For this review, take the finished solid that the model builds, in its own axes (mm). A direction names the side the tool comes from. Coordinates: 2 decimals unless noted, no trailing zeros. Loops run counter-clockwise (first coordinate to the right, second up) from the corner with the lowest first, then second, coordinate; pieces in that order, holes last. Notation, with made-up numbers: M -17.75,57.5 L 41.25,57.5 A21 cw 41.25,93.5 Z; hole C 44.5,14.5 d5. An arc over 180 degrees is marked long. Write item = value, one per line.
from build123d import *

# Parameters (mm, degrees)
F1_R          = 8.89
F1_R_2        = 5.969
F3_R          = 8.89
F3_R_2        = 7.62
F4_DEPTH      = 7.62
F5_DEPTH      = 25.4
F5_DEPTH_BACK = 25.4
F6_R          = 7.62
F7_R          = 7.62
F8_DEPTH      = 25.4
F0_W          = 25.4
F0_H          = 12.7
F9_DEPTH      = 8.89
F9_DEPTH_BACK = 8.89
F10_DEPTH     = 25.4


with BuildPart() as f2:
    # F2: sweep along a path in F0
    with BuildLine(Plane.XY) as f2_path:
        Line((0, 0), (0, 68.940756))
        ThreePointArc((0, 68.940756), (12.7, 81.640756), (25.4, 68.940756))
        Line((25.4, 68.940756), (25.4, 0))
    # F1 (on Front) → F2 (sweep)
    with BuildSketch(Plane.XZ):
        Circle(F1_R)
        Circle(F1_R_2, mode=Mode.SUBTRACT)
    sweep(path=f2_path.line)

    # F3 (on face) → F4 (cut)
    with BuildSketch(Plane.XZ):
        Circle(F3_R)
        Circle(F3_R_2, mode=Mode.SUBTRACT)
        with BuildLine():
            ThreePointArc((34.29, 0), (25.4, 8.89), (16.51, 0))
            ThreePointArc((16.51, 0), (25.4, -8.89), (34.29, 0))
        make_face()
        with BuildLine():
            ThreePointArc((33.02, 0), (25.4, -7.62), (17.78, 0))
            ThreePointArc((17.78, 0), (25.4, 7.62), (33.02, 0))
        make_face(mode=Mode.SUBTRACT)
    extrude(amount=-F4_DEPTH, mode=Mode.SUBTRACT)

    # F0 (on Top) → F5 (cut, two sides)
    with BuildSketch(Plane.XY) as f5_sk:
        with BuildLine():
            Line((-11.195335, 39.121766), (0, 39.121766))
            Line((0, 39.121766), (0, 68.940756))
            ThreePointArc((0, 68.940756), (3.719744, 77.921012), (12.7, 81.640756))
            ThreePointArc((12.7, 81.640756), (21.680256, 77.921012), (25.4, 68.940756))
            Line((25.4, 68.940756), (25.4, 39.121766))
            Line((25.4, 39.121766), (39.424099, 39.121766))
            Line((39.424099, 39.121766), (39.424099, 94.536379))
            Line((39.424099, 94.536379), (-11.195335, 94.536379))
            Line((-11.195335, 94.536379), (-11.195335, 39.121766))
        make_face()
        with BuildLine():
            Line((0, 68.940756), (0, 39.121766))
            Line((0, 39.121766), (12.7, 39.121766))
            Line((12.7, 39.121766), (12.7, 81.640756))
            ThreePointArc((12.7, 81.640756), (3.719744, 77.921012), (0, 68.940756))
        make_face()
        with BuildLine():
            Line((12.7, 39.121766), (25.4, 39.121766))
            Line((25.4, 39.121766), (25.4, 68.940756))
            ThreePointArc((25.4, 68.940756), (21.680256, 77.921012), (12.7, 81.640756))
            Line((12.7, 81.640756), (12.7, 39.121766))
        make_face()
    extrude(amount=F5_DEPTH, mode=Mode.SUBTRACT)
    extrude(f5_sk.sketch, amount=-F5_DEPTH_BACK, mode=Mode.SUBTRACT)

    # F6 (on face) + F7 (on face) → F8 (cut)
    with BuildSketch(Plane(origin=(0, 39.121766, 0), x_dir=(-1, 0, 0), z_dir=(0, 1, 0))):
        Circle(F6_R)
    with BuildSketch(Plane(origin=(0, 39.121766, 0), x_dir=(-1, 0, 0), z_dir=(0, 1, 0))):
        with Locations((-25.4, 0)):
            Circle(F7_R)
    extrude(amount=-F8_DEPTH, mode=Mode.SUBTRACT)

    # F0 (on Top) → F9 (join, two sides)
    with BuildSketch(Plane.XY) as f9_sk:
        with Locations((12.7, 26.517263)):
            Rectangle(F0_W, F0_H)
    extrude(amount=F9_DEPTH)
    extrude(f9_sk.sketch, amount=-F9_DEPTH_BACK)

    # F7 (on face) + F6 (on face) → F10 (cut)
    with BuildSketch(Plane(origin=(0, 39.121766, 0), x_dir=(-1, 0, 0), z_dir=(0, 1, 0))):
        with Locations((-25.4, 0)):
            Circle(F7_R)
    with BuildSketch(Plane(origin=(0, 39.121766, 0), x_dir=(-1, 0, 0), z_dir=(0, 1, 0))):
        Circle(F6_R)
    extrude(amount=-F10_DEPTH, mode=Mode.SUBTRACT)


solid = f2.part
Q1. For pin 1 Ø9 at (x, z) = (25.4, 0) entering from +Y; pin 2 Ø4.5 at (x, z) = (29, -2.5) entering from +Y; pin 3 Ø5 at (x, y) = (24.5, 4.5) entering from -Z; pin 4 Ø5.5 at (x, z) = (13.5, -4) entering from -Y, all flat-tipped, find the tip position at first contact; note any pin that passes through.
Solved:
pin_1 = through
pin_2 = 13.72
pin_3 = -7.62
pin_4 = 20.17
Q2. Draft analysis for pull direction Z (two halves, no side actions). For faces 1 (the face through (31.363, 6.765, -0.262)), 2 (the face through (33.013, 3.757, 0.335)), 3 (the face through (7, 39.122, 4)), state which applies: +Z half, -Z half, draft (parallel to the pull), parting line (faces both ways), or undercut.
Solved:
face_1 = undercut
face_2 = parting line
face_3 = draft
Q3. Add section B-B (x = 27.5). Write out the cut boundary in (y, z), and give its area (3 significant figures).
Solved:
outline = M 0,-7.32 L 7.62,-7.32 L 7.62,-8.64 L 39.12,-8.64 L 39.12,-7.32 L 13.72,-7.32 L 13.72,-5.59 L 0,-5.59 Z; M 0,5.59 L 13.72,5.59 L 13.72,7.32 L 39.12,7.32 L 39.12,8.64 L 7.62,8.64 L 7.62,7.32 L 0,7.32 Z
area = 130 mm²
Q4. For line 1 along Z through (x, y) = (25, 33); line 2 along X through (y, z) = (33, 3.5); line 3 along X through (y, z) = (21, 1.5), list the stretches that pass through material, from the lowest coordinate up.
Solved:
line_1 = -8.88 to -7.61, 7.61 to 8.88
line_2 = -8.17 to -6.77, 6.77 to 8.17, 17.23 to 18.63, 32.17 to 33.57
line_3 = -8.76 to -7.47, 7.47 to 17.93, 32.87 to 34.16
Q5. Add section C-C (z = 0). State how many separate pieces and enclosed holes the cut face has, and give its area (3 significant figures).
Solved:
separate_pieces = 3
enclosed_holes = 0
area = 347 mm²
Q6. Machinability: for faces 4 (the face through (7, 7.62, 4)), 5 (the face through (13, 27, 8.89)), 6 (the face through (33.013, 26.6, 0.335)), which of the approach directions +Z, -Z, +X, -X, +Y, -Y give a long, thin tool a straight path to every point of the face, cutting with its end or side? Answer none if there is none.
Solved:
face_4 = -Y
face_5 = +Z, +X, -X, +Y, -Y
face_6 = +Y
Q7. Add section D-D (y = 4). Write out the cut boundary in (x, z), and give its area (3 significant figures).
Solved:
outline = C 0,0 d15.24; C 25.4,0 d15.24; hole C 0,0 d11.94; hole C 25.4,0 d11.94
area = 141 mm²
Q8. Add section A-A (y = 19.5). Write out the cut boundary in (x, z).
Solved:
outline = C 0,0 d17.78; C 25.4,0 d17.78; hole C 0,0 d15.24; hole C 25.4,0 d15.24
